from build123d import *

# Parameters (mm, degrees)
SKETCH1_R           = 12.5
SKETCH1_R_2         = 1.25
SKETCH1_R_3         = 3
BOSS_EXTRUDE1_DEPTH = 10
FILLET1_R           = 1


with BuildPart() as part:
    # Sketch1 → Boss-Extrude1 (new body)
    with BuildSketch(Plane(origin=(0, 0, 0), x_dir=(1, 0, 0), z_dir=(0, 1, 0))):
        with Locations(Location((0, 0, 0), (0, 0, 270))):
            Circle(SKETCH1_R)
        with Locations(Location((0, 8, 0), (0, 0, 270))):
            Circle(SKETCH1_R_2, mode=Mode.SUBTRACT)
        with Locations(Location((5.656854249, 5.656854249, 0), (0, 0, 270))):
            Circle(SKETCH1_R_2, mode=Mode.SUBTRACT)
        with Locations(Location((0, 0, 0), (0, 0, 270))):
            Circle(SKETCH1_R_3, mode=Mode.SUBTRACT)
        with Locations(Location((8, 0, 0), (0, 0, 270))):
            Circle(SKETCH1_R_2, mode=Mode.SUBTRACT)
        with Locations(Location((5.656854249, -5.656854249, 0), (0, 0, 270))):
            Circle(SKETCH1_R_2, mode=Mode.SUBTRACT)
        with Locations(Location((0, -8, 0), (0, 0, 270))):
            Circle(SKETCH1_R_2, mode=Mode.SUBTRACT)
        with Locations(Location((-5.656854249, -5.656854249, 0), (0, 0, 270))):
            Circle(SKETCH1_R_2, mode=Mode.SUBTRACT)
        with Locations(Location((-8, 0, 0), (0, 0, 270))):
            Circle(SKETCH1_R_2, mode=Mode.SUBTRACT)
        with Locations(Location((-5.656854249, 5.656854249, 0), (0, 0, 270))):
            Circle(SKETCH1_R_2, mode=Mode.SUBTRACT)
    extrude(amount=BOSS_EXTRUDE1_DEPTH)

    # Fillet1
    fillet1_edges = [part.edges().sort_by_distance(p)[0] for p in [
        (0, 0, -12.5),
        (0, 10, -12.5),
    ]]
    fillet(fillet1_edges, radius=FILLET1_R)


solid = part.part
Can you work these out from the model? Positions are in its coordinate system, mm. Coordinates: 2 decimals unless noted, no trailing zeros. Write each loop counter-clockwise with the first axis right and the second up, starting at its lowest first coordinate (ties: lowest second). Pieces come first, ordered by that corner, then holes. Notation, with made-up numbers: (57.5, 58) - (97.5, 58) arc R21 ccw to (97.5, 69) - close; hole circle Ø6 at (58.5, 58.5). An arc over 180 degrees is marked (long way). Return JSON: item names as keys, results as strings. Group by question number.
Item 1: If we section it at B-B (z = 0): Write out the boundary of the cut face in (x, y), then the cut area to 3 significant figures.
Item 2: If we section it at C-C (y = 7.25): Count the separate pieces of the cut face and the enclosed holes in it, then the cut area to 3 significant figures.
Item 3: Please list where these lines run through material, in increasing order: probe 1 along X at (y, z) = (2.5, 0); probe 2 along X at (y, z) = (5.75, 1); probe 3 along X at (y, z) = (6.25, -6.25).
Item 4: We'd pull the mould along X, two halves only. Please class faces 1 (the face through (0.9, 4.93, 2.86)), 2 (the face through (3.755, 4.944, 11.923)), 3 (the face through (-2.4, 0, 2.4)), 4 (the face through (0.05, 4.93, 6.75)): pulls with the +X half, pulls with the -X half, needs draft (parallel to the pull), parting line crosses it, or undercut.
Item 5: If we section it at A-A (x = 0): Write out the boundary of the cut face in (y, z).
Item 6: I'm going to push a flat-ended pin straight in: pin 1 Ø1 at (y, z) = (6, 8.5) entering from +X. Where does the tip first touch, or does it pass through?
Return value:
{
 "1": {"outline": "(-12.5, 1) arc R1 ccw to (-11.5, 0) - (-9.25, 0) - (-9.25, 10) - (-11.5, 10) arc R1 ccw to (-12.5, 9) - close; (-6.75, 0) - (-3, 0) - (-3, 10) - (-6.75, 10) - close; (3, 0) - (6.75, 0) - (6.75, 10) - (3, 10) - close; (9.25, 0) - (11.5, 0) arc R1 ccw to (12.5, 1) - (12.5, 9) arc R1 ccw to (11.5, 10) - (9.25, 10) - close", "area": "139 mm^2"},
 "2": {"separate pieces": "1", "enclosed holes": "9", "area": "423 mm^2"},
 "3": {"probe 1": "x = -12.5 to -9.25, -6.75 to -3, 3 to 6.75, 9.25 to 12.5", "probe 2": "x = -12.46 to -8.75, -7.25 to -2.83, 2.83 to 7.25, 8.75 to 12.46", "probe 3": "x = -10.83 to -6.76, -4.56 to 4.56, 6.76 to 10.83"},
 "4": {"face 1": "undercut", "face 2": "parting line crosses it", "face 3": "needs draft", "face 4": "undercut"},
 "5": {"outline": "(0, -11.5) arc R1 ccw to (1, -12.5) - (9, -12.5) arc R1 ccw to (10, -11.5) - (10, -9.25) - (0, -9.25) - close; (0, -6.75) - (10, -6.75) - (10, -3) - (0, -3) - close; (0, 3) - (10, 3) - (10, 6.75) - (0, 6.75) - close; (0, 9.25) - (10, 9.25) - (10, 11.5) arc R1 ccw to (9, 12.5) - (1, 12.5) arc R1 ccw to (0, 11.5) - close"},
 "6": {"pin 1": "stops at x = 9.6"}
}
